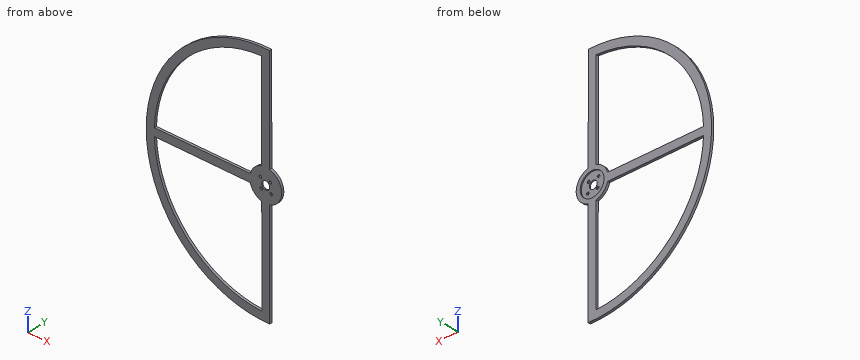
from build123d import *

# Parameters (mm, degrees)
SKETCH1_R           = 5
SKETCH1_R_2         = 1.7
BOSS_EXTRUDE1_DEPTH = 3
SKETCH2_R           = 15
CUT_EXTRUDE1_DEPTH  = 1.5


with BuildPart() as part:
    # Sketch1 → Boss-Extrude1 (new body)
    with BuildSketch(Plane(origin=(0, 0, 0), x_dir=(1, 0, 0), z_dir=(0, 1, 0))):
        with BuildLine():
            Line((5, -19.364916731), (4.6875, -149.926739922))
            ThreePointArc((4.6875, -149.926739922), (-149.999918535, 0.156331529), (5, 149.916643506))
            Line((5, 149.916643506), (5, 19.364916731))
            ThreePointArc((5, 19.364916731), (20, 0), (5, -19.364916731))
        make_face()
        Circle(SKETCH1_R, mode=Mode.SUBTRACT)
        with Locations((-5.656854249, 5.656854249)):
            Circle(SKETCH1_R_2, mode=Mode.SUBTRACT)
        with Locations((5.656854249, -5.656854249)):
            Circle(SKETCH1_R_2, mode=Mode.SUBTRACT)
        with Locations((6.717514421, 6.717514421)):
            Circle(SKETCH1_R_2, mode=Mode.SUBTRACT)
        with Locations((-6.717514421, -6.717514421)):
            Circle(SKETCH1_R_2, mode=Mode.SUBTRACT)
        with BuildLine():
            Line((-5, -19.364916731), (-5, -139.910685796))
            ThreePointArc((-5, -139.910685796), (-98.994949366, -98.994949366), (-139.910685796, -5))
            Line((-139.910685796, -5), (-19.364916731, -5))
            ThreePointArc((-19.364916731, -5), (-14.142135624, -14.142135624), (-5, -19.364916731))
        make_face(mode=Mode.SUBTRACT)
        with BuildLine():
            Line((-5, 19.364916731), (-4.666666667, 139.922200605))
            ThreePointArc((-4.666666667, 139.922200605), (-98.994949366, 98.994949366), (-139.922200605, 4.666666667))
            Line((-139.922200605, 4.666666667), (-19.364916731, 5))
            ThreePointArc((-19.364916731, 5), (-14.142135624, 14.142135624), (-5, 19.364916731))
        make_face(mode=Mode.SUBTRACT)
    extrude(amount=BOSS_EXTRUDE1_DEPTH)

    # Sketch2 → Cut-Extrude1 (cut)
    with BuildSketch(Plane(origin=(0, 3, 0), x_dir=(1, 0, 0), z_dir=(0, 1, 0))):
        Circle(SKETCH2_R)
    extrude(amount=-CUT_EXTRUDE1_DEPTH, mode=Mode.SUBTRACT)


solid = part.part
The listing builds one solid part. Answer for the finished solid, in the listing's coordinates (mm). Round coordinates to 2 decimals unless told otherwise and drop trailing zeros. Order: outer loops, then holes, each group sorted by start corner. A loop starts at its lowest first (then second) coordinate and runs counter-clockwise, first axis right, second up. Notation, with made-up numbers: (-2, 41.5) -> (40, 41.5) arc R13 ccw to (40, 60.5) -> close; hole circle Ø6 at (55, -36). An arc over 180 degrees is marked (long way). Put each result on its own line as item: value.
Q1. Section B-B, the plane x = 0 is taken. Write down the section's boundary in (y, z), and give its area (3 significant figures).
Results list:
outline: (0, -150) -> (3, -150) -> (3, -15) -> (1.5, -15) -> (1.5, -5) -> (0, -5) -> close; (0, 5) -> (1.5, 5) -> (1.5, 15) -> (3, 15) -> (3, 150) -> (0, 150) -> close
area: 840 mm^2
Q2. Consider line 1 along Z through (x, y) = (-58, 0.45); line 2 along Z through (x, y) = (-103, 0.25); line 3 along Z through (x, y) = (0, 1.9). Determine where each line is inside the solid, lowest interval first.
Results list:
line 1: -138.33 to -127.42, -4.89 to 5, 127.42 to 138.33
line 2: -109.05 to -94.82, -4.77 to 5, 94.82 to 109.05
line 3: -150 to -15, 15 to 150
Q3. Each of these flat-tipped pins is pushed along its axis until it touches: P1, Ø4.5, axis at x = 6.72, z = -6.72, coming from the +Y side; P2, Ø2, axis at x = -6.72, z = 6.72, coming from the +Y side; P3, Ø0.9, axis at y = 2, z = 57.5, coming from the -X side; P4, Ø1, axis at x = -60, y = 1.5, coming from the +Z side. Where does it stop, or does it pass through?
Results list:
P1: y = 1.5
P2: through
P3: x = -138.73
P4: z = 137.69
Q4. Section A-A, the plane z = 0 is taken. Write down the section's boundary in (x, y), and give its area (3 significant figures).
Results list:
outline: (-150, 0) -> (-5, 0) -> (-5, 1.5) -> (-15, 1.5) -> (-15, 3) -> (-150, 3) -> close; (5, 0) -> (20, 0) -> (20, 3) -> (15, 3) -> (15, 1.5) -> (5, 1.5) -> close
area: 450 mm^2
Q5. Section C-C, the plane y = 2.25 is taken. Write down the section's boundary in (x, z), and give its area (3 significant figures).
Results list:
outline: (4.69, 149.93) arc R150 ccw (long way) to (5, -149.92) -> (5, -19.36) arc R20 ccw to (5, 19.36) -> close; hole (-139.92, -4.67) arc R140 ccw to (-4.67, -139.92) -> (-5, -19.36) arc R20 cw to (-19.36, -5) -> close; hole (-139.91, 5) -> (-19.36, 5) arc R20 cw to (-5, 19.36) -> (-5, 139.91) arc R140 ccw to start; hole circle Ø30 at (0, 0)
area: 8,750 mm^2
Q6. Section D-D, the plane x = -100.5 is taken. Write down the section's boundary in (y, z).
Results list:
outline: (0, -111.35) -> (3, -111.35) -> (3, -97.47) -> (0, -97.47) -> close; (0, -4.78) -> (3, -4.78) -> (3, 5) -> (0, 5) -> close; (0, 97.47) -> (3, 97.47) -> (3, 111.35) -> (0, 111.35) -> close
